```python
from build123d import *

# Parameters (mm, degrees)
SKETCH1_W                = 38.1
SKETCH1_H                = 31.75
BOSS_EXTRUDE1_DEPTH      = 5.8
SKETCH2_R                = 8
CUT_EXTRUDE1_DEPTH       = 50.933080217
M3_CLEARANCE_HOLE1_D     = 3.4
M3_CLEARANCE_HOLE1_DEPTH = 6.35
M3_CLEARANCE_HOLE1_TIP   = 1.021463052
M3_CLEARANCE_HOLE2_D     = 3.4
M3_CLEARANCE_HOLE2_DEPTH = 6.35
M3_CLEARANCE_HOLE2_TIP   = 1.021463052
FILLET1_R                = 3.175


with BuildPart() as part:
    # Sketch1 → Boss-Extrude1 (new body)
    with BuildSketch(Plane.XY):
        with Locations((19.05, 15.875)):
            Rectangle(SKETCH1_W, SKETCH1_H)
    extrude(amount=BOSS_EXTRUDE1_DEPTH)

    # Sketch2 → Cut-Extrude1 (cut, through all)
    with BuildSketch(Plane.XY.offset(5.8)):
        with Locations((19.05, 15.875)):
            Circle(SKETCH2_R)
    extrude(amount=-CUT_EXTRUDE1_DEPTH, mode=Mode.SUBTRACT)

    # M3 Clearance Hole1
    with Locations(Plane.XY.offset(5.8)):
        with Locations((30.05, 15.875), (24.55, 25.401279442), (13.55, 25.401279442), (8.05, 15.875), (13.55, 6.348720558), (24.55, 6.348720558)):
            Hole(M3_CLEARANCE_HOLE1_D / 2, depth=M3_CLEARANCE_HOLE1_DEPTH)
            with Locations((0, 0, -(M3_CLEARANCE_HOLE1_DEPTH + M3_CLEARANCE_HOLE1_TIP / 2))):  # 118° drill point
                Cone(0, M3_CLEARANCE_HOLE1_D / 2, M3_CLEARANCE_HOLE1_TIP, mode=Mode.SUBTRACT)

    # M3 Clearance Hole2
    with Locations(Plane.XY.offset(5.8)):
        with Locations((3.175, 28.575), (34.925, 28.575), (34.925, 3.175), (3.175, 3.175)):
            Hole(M3_CLEARANCE_HOLE2_D / 2, depth=M3_CLEARANCE_HOLE2_DEPTH)
            with Locations((0, 0, -(M3_CLEARANCE_HOLE2_DEPTH + M3_CLEARANCE_HOLE2_TIP / 2))):  # 118° drill point
                Cone(0, M3_CLEARANCE_HOLE2_D / 2, M3_CLEARANCE_HOLE2_TIP, mode=Mode.SUBTRACT)

    # Fillet1
    fillet1_edges = [part.edges().sort_by_distance(p)[0] for p in [
        (0, 31.75, 2.9),
        (38.1, 31.75, 2.9),
        (38.1, 0, 2.9),
        (0, 0, 2.9),
    ]]
    fillet(fillet1_edges, radius=FILLET1_R)


solid = part.part
```
Input: part model. Units: mm. Frame: model coordinates. Round coordinates to 2 decimals unless told otherwise and drop trailing zeros. Loops run counter-clockwise (first coordinate to the right, second up) from the corner with the lowest first, then second, coordinate; pieces in that order, holes last. Notation, with made-up numbers: (49.5, -7.5) -> (63.5, -7.5) arc R15 cw to (63.5, 1.5) -> close; hole circle Ø11 at (61, 21). An arc over 180 degrees is marked (long way). One line per item, written item: value.
(1) Material intervals for line 1 (X direction, y = 25.5, z = 2.4); line 2 (Y direction, x = 35, z = 1.5); line 3 (Y direction, x = 19, z = 1), sorted ascending. Write a range as [from, to].
Geometry check:
line 1: [0, 11.85], [15.25, 22.85], [26.25, 38.1]
line 2: [0, 1.48], [4.87, 26.88], [30.27, 31.75]
line 3: [0, 7.88], [23.87, 31.75]
(2) Section C-C (x = 35.5). Return the cut outline in (y, z).
Geometry check:
outline: (0.05, 0) -> (1.58, 0) -> (1.58, 5.8) -> (0.05, 5.8) -> close; (4.77, 0) -> (26.98, 0) -> (26.98, 5.8) -> (4.77, 5.8) -> close; (30.17, 0) -> (31.7, 0) -> (31.7, 5.8) -> (30.17, 5.8) -> close
(3) Section D-D (y = 8.5). Return the cut outline in (x, z), plus the area to 3 significant figures.
Geometry check:
outline: (0, 0) -> (15.95, 0) -> (15.95, 5.8) -> (0, 5.8) -> close; (22.15, 0) -> (38.1, 0) -> (38.1, 5.8) -> (22.15, 5.8) -> close
area: 185 mm2
(4) Mould query, pull axis Y, two halves, no side actions, for faces 1 (the face through (19, 0, 3)), 2 (the face through (13.771, 8.034, 2.859)), 3 (the face through (0, 16, 3)). Classes: pulls with the +Y half, pulls with the -Y half, needs draft (parallel to the pull), parting line crosses it, or undercut.
Geometry check:
face 1: pulls with the -Y half
face 2: undercut
face 3: needs draft
(5) Section B-B (y = 4). Return the cut outline in (x, z), plus the area to 3 significant figures.
Geometry check:
outline: (0, 0) -> (1.69, 0) -> (1.69, 5.8) -> (0, 5.8) -> close; (4.66, 0) -> (33.44, 0) -> (33.44, 5.8) -> (4.66, 5.8) -> close; (36.41, 0) -> (38.1, 0) -> (38.1, 5.8) -> (36.41, 5.8) -> close
area: 186 mm2
(6) Pin query (flat end, axial travel): pin 1 (2.5 mm diameter, centred on x = 8.05, y = 15.875, fed in from -Z). Return the tip coordinate at first contact, or that it passes through.
Geometry check:
pin 1: through
(7) Section A-A (x = 30.05). Return the cut outline in (y, z) (3 decimals), plus the area to 3 significant figures.
Geometry check:
outline: (0, 0) -> (14.175, 0) -> (14.175, 5.8) -> (0, 5.8) -> close; (17.575, 0) -> (31.75, 0) -> (31.75, 5.8) -> (17.575, 5.8) -> close
area: 164 mm2
